Design review of the part built by this model. Coordinates are the model's own, in mm. A direction names the side the tool comes from. Round coordinates to 2 decimals unless told otherwise and drop trailing zeros. Loops run counter-clockwise (first coordinate to the right, second up) from the corner with the lowest first, then second, coordinate; pieces in that order, holes last. Notation, with made-up numbers: M -0.75,57.5 L 7.25,57.5 A12 cw 7.25,71.5 Z; hole C 32.5,36.25 d6. An arc over 180 degrees is marked long. Answer as CSV lines item,"result". Start each with the question number.
from build123d import *

# Parameters (mm, degrees)
SKETCH3_R           = 25
BOSS_EXTRUDE2_DEPTH = 30
CUT_EXTRUDE1_DEPTH  = 15
SKETCH6_W           = 60
SKETCH6_H           = 65
BOSS_EXTRUDE3_DEPTH = 2


with BuildPart() as part:
    # Sketch3 → Boss-Extrude2 (new body)
    with BuildSketch(Plane(origin=(0, 0, 0), x_dir=(0, 0, -1), z_dir=(1, 0, 0))):
        Circle(SKETCH3_R)
    extrude(amount=BOSS_EXTRUDE2_DEPTH)

    # Sketch4 → Cut-Extrude1 (cut)
    with BuildSketch(Plane(origin=(30, 0, 0), x_dir=(0, 0, -1), z_dir=(1, 0, 0))):
        with BuildLine():
            Line((6.3, 3.252817327), (22.023267424, 1.812565295))
            ThreePointArc((22.023267424, 1.812565295), (23.090240495, 0.619111869), (21.975368687, -0.529723832))
            Line((21.975368687, -0.529723832), (6.3, -3.196442617))
            Line((6.3, -3.196442617), (6.3, -16.25))
            Line((6.3, -16.25), (-6.3, -16.25))
            Line((-6.3, -16.25), (-6.3, 16.25))
            Line((-6.3, 16.25), (6.3, 16.25))
            Line((6.3, 16.25), (6.3, 3.252817327))
        make_face()
    extrude(amount=-CUT_EXTRUDE1_DEPTH, mode=Mode.SUBTRACT)

    # Sketch6 → Boss-Extrude3 (add)
    with BuildSketch(Plane.ZY):
        Rectangle(SKETCH6_W, SKETCH6_H)
    extrude(amount=BOSS_EXTRUDE3_DEPTH)


solid = part.part
Item 1: The part is to be moulded in two halves that separate along Z. For faces 1 (the face through (14.79, 7.509, -23.846)), 2 (the face through (-1, 0, -30)), 3 (the face through (-1, 32.5, 0)), 4 (the face through (23, 10, -6.3)), say which applies: +Z half, -Z half, draft (parallel to the pull), parting line (faces both ways), or undercut.
Item 2: Consider section B-B, the plane x = 17.5. Write out the cut boundary in (y, z).
Item 3: To check wall thickness, follow line 1 (X direction, y = -13.5, z = 26); line 2 (X direction, y = -10.5, z = 5); line 3 (Z direction, x = 27, y = -3.5). State the ranges of each line that lie inside material, in increasing order.
Item 4: Consider section D-D, the plane x = 13.5. Write out the cut boundary in (y, z).
Item 5: Consider section A-A, the plane z = 0. Write out the cut boundary in (x, y), then the cut area to 3 significant figures.
Item 6: Consider section C-C, the plane y = 19. Write out the cut boundary in (x, z), then the cut area to 3 significant figures.
Item 7: Tool access review of faces 5 (the face through (-2, 0, 0)), 6 (the face through (23, -16.25, 0)): name each direction out of +Z, -Z, +X, -X, +Y, -Y from which nothing blocks a thin tool from reaching the whole face with its end or side.
Item 8: Insertion check: pin 1 Ø10 at (x, z) = (23.5, -2) entering from -Y; pin 2 Ø7.5 at (x, y) = (20, -8) entering from -Z; pin 3 Ø8 at (x, z) = (3, 22.5) entering from +Y; pin 4 Ø1 at (x, y) = (7, 8) entering from +Z. Each pin has a flat end and moves straight along its axis. Give the tip position at first contact, or say it passes through.
Found:
1,face 1,"parting line"
1,face 2,"-Z half"
1,face 3,"draft"
1,face 4,"undercut"
2,outline,"C 0,0 d50; hole M -16.25,-6.3 L -3.2,-6.3 L -0.53,-21.98 A1.17 ccw 1.81,-22.02 L 3.25,-6.3 L 16.25,-6.3 L 16.25,6.3 L -16.25,6.3 Z"
3,line 1,"x = -2 to 0"
3,line 2,"x = -2 to 15"
3,line 3,"z = -24.75 to -6.3, 6.3 to 24.75"
4,outline,"C 0,0 d50"
5,outline,"M -2,-32.5 L 0,-32.5 L 0,-25 L 30,-25 L 30,-16.25 L 15,-16.25 L 15,16.25 L 30,16.25 L 30,25 L 0,25 L 0,32.5 L -2,32.5 Z"
5,area,"1,140 mm^2"
6,outline,"M -2,-30 L 0,-30 L 0,-16.25 L 30,-16.25 L 30,16.25 L 0,16.25 L 0,30 L -2,30 Z"
6,area,"1,090 mm^2"
7,face 5,"+Z, -Z, -X, +Y, -Y"
7,face 6,"+X"
8,pin 1,"stops at y = -25"
8,pin 2,"stops at z = -24.64"
8,pin 3,"stops at y = 32.5"
8,pin 4,"stops at z = 23.85"
